```python
from build123d import *
from build123d.topology import SkipClean

# Parameters (mm, degrees)
BOSS_EXTRUDE1_DEPTH   = 67.5
BOSS_EXTRUDE1_2_DEPTH = 67.5
BOSS_EXTRUDE1_3_DEPTH = 67.5
BOSS_EXTRUDE1_4_DEPTH = 67.5
BOSS_EXTRUDE1_5_DEPTH = 67.5
BOSS_EXTRUDE1_6_DEPTH = 67.5
BOSS_EXTRUDE2_START   = -2.5
SKETCH2_R             = 55
SKETCH2_R_2           = 40
BOSS_EXTRUDE2_DEPTH   = 2.5
BOSS_EXTRUDE3_START   = 67.5
SKETCH3_R             = 55
SKETCH3_R_2           = 7.5
BOSS_EXTRUDE3_DEPTH   = 5
SKETCH4_R             = 15
SKETCH4_R_2           = 7.5
BOSS_EXTRUDE4_DEPTH   = 25


with BuildPart() as part:
    # Sketch1 → Boss-Extrude1 (new body)
    with BuildSketch(Plane(origin=(0, 0, 0), x_dir=(1, 0, 0), z_dir=(0, 1, 0))):
        with BuildLine():
            Line((55, 0), (30, 0))
            Line((30, 0), (30, 2.5))
            Line((30, 2.5), (52.941004902, 2.5))
            ThreePointArc((52.941004902, 2.5), (52.137315312, 9.523673244), (50.405995364, 16.377900702))
            Line((50.405995364, 16.377900702), (52.308108396, 16.995934691))
            ThreePointArc((52.308108396, 16.995934691), (54.322858733, 8.603895577), (55, 0))
        make_face()
    extrude(amount=BOSS_EXTRUDE1_DEPTH)



with BuildPart() as body_2:
    # Sketch1 → Boss-Extrude1 2 (new body)
    with BuildSketch(Plane(origin=(0, 0, 0), x_dir=(1, 0, 0), z_dir=(0, 1, 0))):
        with BuildLine():
            Line((27.5, -47.631397208), (15, -25.980762114))
            Line((15, -25.980762114), (17.165063509, -24.730762114))
            Line((17.165063509, -24.730762114), (28.63556596, -44.598255147))
            ThreePointArc((28.63556596, -44.598255147), (34.316400623, -40.390402923), (39.38667575, -35.463922137))
            Line((39.38667575, -35.463922137), (40.872965401, -36.80218335))
            ThreePointArc((40.872965401, -36.80218335), (34.612621508, -42.74302788), (27.5, -47.631397208))
        make_face()
    extrude(amount=BOSS_EXTRUDE1_2_DEPTH)


with BuildPart() as body_3:
    # Sketch1 → Boss-Extrude1 3 (new body)
    with BuildSketch(Plane(origin=(0, 0, 0), x_dir=(1, 0, 0), z_dir=(0, 1, 0))):
        with BuildLine():
            Line((-27.5, -47.631397208), (-15, -25.980762114))
            Line((-15, -25.980762114), (-12.834936491, -27.230762114))
            Line((-12.834936491, -27.230762114), (-24.305438941, -47.098255147))
            ThreePointArc((-24.305438941, -47.098255147), (-17.820914689, -49.914076167), (-11.019319613, -51.841822839))
            Line((-11.019319613, -51.841822839), (-11.435142995, -53.79811804))
            ThreePointArc((-11.435142995, -53.79811804), (-19.710237225, -51.346923457), (-27.5, -47.631397208))
        make_face()
    extrude(amount=BOSS_EXTRUDE1_3_DEPTH)


with BuildPart() as body_4:
    # Sketch1 → Boss-Extrude1 4 (new body)
    with BuildSketch(Plane(origin=(0, 0, 0), x_dir=(1, 0, 0), z_dir=(0, 1, 0))):
        with BuildLine():
            Line((-55, 0), (-30, 0))
            Line((-30, 0), (-30, -2.5))
            Line((-30, -2.5), (-52.941004902, -2.5))
            ThreePointArc((-52.941004902, -2.5), (-52.137315312, -9.523673244), (-50.405995364, -16.377900702))
            Line((-50.405995364, -16.377900702), (-52.308108396, -16.995934691))
            ThreePointArc((-52.308108396, -16.995934691), (-54.322858733, -8.603895577), (-55, 0))
        make_face()
    extrude(amount=BOSS_EXTRUDE1_4_DEPTH)


with BuildPart() as body_5:
    # Sketch1 → Boss-Extrude1 5 (new body)
    with BuildSketch(Plane(origin=(0, 0, 0), x_dir=(1, 0, 0), z_dir=(0, 1, 0))):
        with BuildLine():
            Line((-27.5, 47.631397208), (-15, 25.980762114))
            Line((-15, 25.980762114), (-17.165063509, 24.730762114))
            Line((-17.165063509, 24.730762114), (-28.63556596, 44.598255147))
            ThreePointArc((-28.63556596, 44.598255147), (-34.316400623, 40.390402923), (-39.38667575, 35.463922137))
            Line((-39.38667575, 35.463922137), (-40.872965401, 36.80218335))
            ThreePointArc((-40.872965401, 36.80218335), (-34.612621508, 42.74302788), (-27.5, 47.631397208))
        make_face()
    extrude(amount=BOSS_EXTRUDE1_5_DEPTH)


with BuildPart() as body_6:
    # Sketch1 → Boss-Extrude1 6 (new body)
    with BuildSketch(Plane(origin=(0, 0, 0), x_dir=(1, 0, 0), z_dir=(0, 1, 0))):
        with BuildLine():
            Line((27.5, 47.631397208), (15, 25.980762114))
            Line((15, 25.980762114), (12.834936491, 27.230762114))
            Line((12.834936491, 27.230762114), (24.305438941, 47.098255147))
            ThreePointArc((24.305438941, 47.098255147), (17.820914689, 49.914076167), (11.019319613, 51.841822839))
            Line((11.019319613, 51.841822839), (11.435142995, 53.79811804))
            ThreePointArc((11.435142995, 53.79811804), (19.710237225, 51.346923457), (27.5, 47.631397208))
        make_face()
    extrude(amount=BOSS_EXTRUDE1_6_DEPTH)


with BuildPart() as part_1:
    add(part.part)

    add(body_2.part)  # Boss-Extrude2 merges body 2

    add(body_3.part)  # Boss-Extrude2 merges body 3

    add(body_4.part)  # Boss-Extrude2 merges body 4

    add(body_5.part)  # Boss-Extrude2 merges body 5

    add(body_6.part)  # Boss-Extrude2 merges body 6
    # Sketch2 → Boss-Extrude2 (add)
    with BuildSketch(Plane(origin=(0, 0, 0), x_dir=(1, 0, 0), z_dir=(0, 1, 0)).offset(BOSS_EXTRUDE2_START)):
        with Locations(Location((0, 0, 0), (0, 0, 78))):
            Circle(SKETCH2_R)
        with Locations(Location((0, 0, 0), (0, 0, 270))):
            Circle(SKETCH2_R_2, mode=Mode.SUBTRACT)
    extrude(amount=BOSS_EXTRUDE2_DEPTH)

    # Sketch3 → Boss-Extrude3 (add)
    with SkipClean():  # the faces are left unmerged after this step: merging them gives an invalid solid
        with BuildSketch(Plane(origin=(0, 0, 0), x_dir=(1, 0, 0), z_dir=(0, 1, 0)).offset(BOSS_EXTRUDE3_START)):
            with Locations(Location((0, 0, 0), (0, 0, 270))):
                Circle(SKETCH3_R)
            with Locations(Location((0, 0, 0), (0, 0, 270))):
                Circle(SKETCH3_R_2, mode=Mode.SUBTRACT)
        extrude(amount=BOSS_EXTRUDE3_DEPTH)

    # Sketch4 → Boss-Extrude4 (add)
    with SkipClean():  # the faces are left unmerged after this step: merging them gives an invalid solid
        with BuildSketch(Plane(origin=(0, 72.5, 0), x_dir=(1, 0, 0), z_dir=(0, 1, 0))):
            with Locations(Location((0, 0, 0), (0, 0, 270))):
                Circle(SKETCH4_R)
            with Locations(Location((0, 0, 0), (0, 0, 270))):
                Circle(SKETCH4_R_2, mode=Mode.SUBTRACT)
        extrude(amount=BOSS_EXTRUDE4_DEPTH)


solid = part_1.part
```
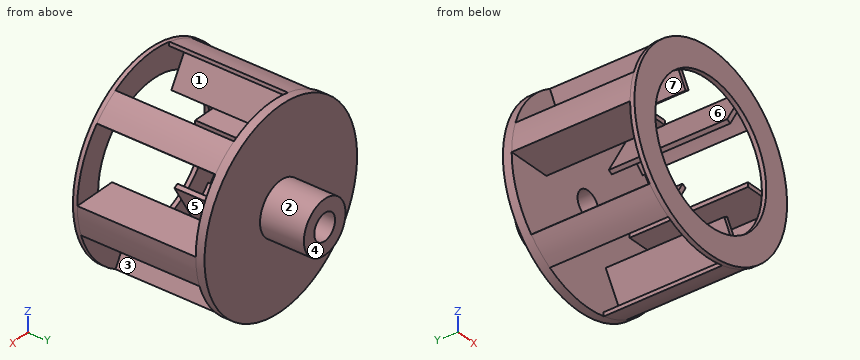
Check sheet for the modelled part. Datum: model origin and axes. Units: mm. Face numbers are marked on the shaded views. A direction names the side the tool comes from. Coordinates: 2 decimals unless noted, no trailing zeros. Order: outer loops, then holes, each group sorted by start corner. A loop starts at its lowest first (then second) coordinate and runs counter-clockwise, first axis right, second up. Notation, with made-up numbers: (-38, 36) -> (15, 36) arc R16 cw to (15, 50) -> close; hole circle Ø11 at (14.25, -14). An arc over 180 degrees is marked (long way). Write item = value, one per line. Start each with the question number.
1) Mould release check, pull along Z, two halves, no side actions. Record for the marked faces 4, 5, 6 and 7: +Z half, -Z half, draft (parallel to the pull), parting line (faces both ways), or undercut.
2) Go/stop test with flat-tipped pins: P1, Ø6, axis at y = 15.5, z = -8.5, coming from the +X side; P2, Ø12, axis at y = 56.5, z = 20, coming from the -X side; P3, Ø18.5, axis at x = -46, y = 44.5, coming from the +Z side; P4, Ø17, axis at x = 0, z = 0, coming from the +Y side. Record where each tip stops, or that it passes through.
3) Access from +Z, -Z, +X, -X, +Y, -Y to the whole of each face (thin tool, end or side, straight path). Record for the marked faces 1, 2 and 3.
4) Cross-section at A-A (x = 0). Enter the section's corners in (y, z), then the cut area to 3 significant figures.
5) Material ranges on L1, parallel to X at y = 77, z = 0; L2, parallel to Z at x = 0, y = -1; L3, parallel to Y at x = -44, z = 18.5, recorded low to high.
6) Cross-section at B-B (z = 22.5). Enter the section's corners in (x, y).
7) Cross-section at D-D (y = 57). State how many separate pieces and enclosed holes the cut face has, then the cut area to 3 significant figures.
8) Cross-section at C-C (x = -26). Enter the section's corners in (y, z).
Ans:
q1.face_4 = draft
q1.face_5 = -Z half
q1.face_6 = +Z half
q1.face_7 = undercut
q2.P1 = 54.72
q2.P2 = -53.19
q2.P3 = 17
q2.P4 = 97.5
q3.face_1 = none
q3.face_2 = +Y
q3.face_3 = +X
q4.outline = (-2.5, -55) -> (0, -55) -> (0, -40) -> (-2.5, -40) -> close; (-2.5, 40) -> (0, 40) -> (0, 55) -> (-2.5, 55) -> close; (67.5, -55) -> (72.5, -55) -> (72.5, -15) -> (97.5, -15) -> (97.5, -7.5) -> (67.5, -7.5) -> close; (67.5, 7.5) -> (97.5, 7.5) -> (97.5, 15) -> (72.5, 15) -> (72.5, 55) -> (67.5, 55) -> close
q4.area = 925 mm²
q5.L1 = -15 to -7.5, 7.5 to 15
q5.L2 = -55 to -40, 40 to 55
q5.L3 = -2.5 to 0, 67.5 to 72.5
q6.outline = (-50.19, -2.5) -> (-33.07, -2.5) -> (-33.07, 0) -> (-50.19, 0) -> close; (-50.19, 67.5) -> (50.19, 67.5) -> (50.19, 72.5) -> (-50.19, 72.5) -> close; (33.07, -2.5) -> (50.19, -2.5) -> (50.19, 0) -> (33.07, 0) -> close
q7.separate_pieces = 6
q7.enclosed_holes = 0
q7.area = 548 mm²
q8.outline = (-2.5, -48.47) -> (0, -48.47) -> (0, -45.03) -> (67.5, -45.03) -> (67.5, -48.47) -> (72.5, -48.47) -> (72.5, 48.47) -> (-2.5, 48.47) -> (-2.5, 30.4) -> (0, 30.4) -> (0, 45.03) -> (67.5, 45.03) -> (67.5, -40.03) -> (0, -40.03) -> (0, -30.4) -> (-2.5, -30.4) -> close
